```python
from build123d import *

# Parameters (mm, degrees)
SKETCH_1_W               = 26.5
SKETCH_1_H               = 26.5
SKETCH_1_R               = 9.25
EXTRUDE_1_DEPTH          = 7.5
SKETCH_3_R               = 1.75
CUT_EXTRUDE_1_DEPTH      = 14.25
CUT_EXTRUDE_1_DEPTH_BACK = 14.25


with BuildPart() as part:
    # ｽｹｯﾁ1 → ﾎﾞｽ - 押し出し1 (new body, symmetric)
    with BuildSketch(Plane.XY):
        Rectangle(SKETCH_1_W, SKETCH_1_H)
        Circle(SKETCH_1_R, mode=Mode.SUBTRACT)
    extrude(amount=EXTRUDE_1_DEPTH, both=True)

    # ｽｹｯﾁ3 → ｶｯﾄ - 押し出し1 (cut, two sides)
    with BuildSketch(Plane(origin=(0, 0, 0), x_dir=(0, 0, -1), z_dir=(1, 0, 0))) as cut_extrude_1_sk:
        Circle(SKETCH_3_R)
    extrude(amount=CUT_EXTRUDE_1_DEPTH, mode=Mode.SUBTRACT)
    extrude(cut_extrude_1_sk.sketch, amount=-CUT_EXTRUDE_1_DEPTH_BACK, mode=Mode.SUBTRACT)


solid = part.part
```
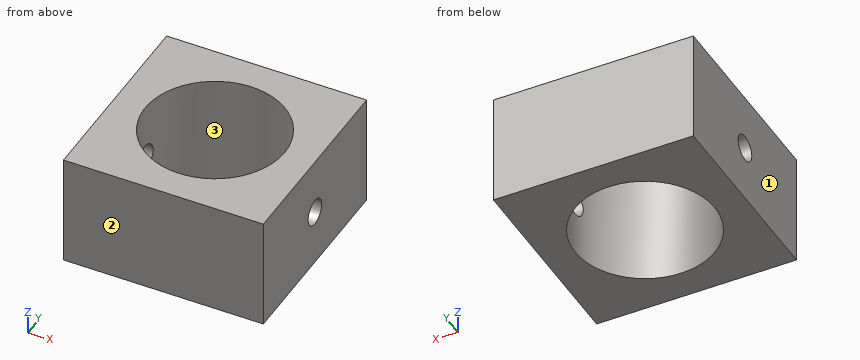
Could you check a few things on this model? Use its own coordinates, in mm. Face numbers are marked on the shaded views. Round coordinates to 2 decimals unless told otherwise and drop trailing zeros. Loops run counter-clockwise (first coordinate to the right, second up) from the corner with the lowest first, then second, coordinate; pieces in that order, holes last. Notation, with made-up numbers: (47.25, 74.5) - (56.25, 74.5) arc R14 cw to (56.25, 93.5) - close; hole circle Ø1 at (-11, 44). An arc over 180 degrees is marked (long way). Answer as CSV lines item,"result".
1. I want a section at C-C on x = 10. List the corners of the cut face in (y, z) for me, then the cut area to 3 significant figures.
Filled in:
outline,"(-13.25, -7.5) - (13.25, -7.5) - (13.25, 7.5) - (-13.25, 7.5) - close; hole circle Ø3.5 at (0, 0)"
area,"388 mm^2"
2. I want a section at B-B on y = 0. List the corners of the cut face in (x, z) for me, then the cut area to 3 significant figures.
Filled in:
outline,"(-13.25, -7.5) - (-9.25, -7.5) - (-9.25, -1.75) - (-13.25, -1.75) - close; (-13.25, 1.75) - (-9.25, 1.75) - (-9.25, 7.5) - (-13.25, 7.5) - close; (9.25, -7.5) - (13.25, -7.5) - (13.25, -1.75) - (9.25, -1.75) - close; (9.25, 1.75) - (13.25, 1.75) - (13.25, 7.5) - (9.25, 7.5) - close"
area,"92.0 mm^2"
3. Please list where these lines run through material, in increasing order: line 1 along Y through (x, z) = (0, 3.5); line 2 along Y through (x, z) = (-12.4, 0); line 3 along Z through (x, y) = (12.15, 0). Write a range as [from, to].
Filled in:
line 1,"y = [-13.25, -9.25], [9.25, 13.25]"
line 2,"y = [-13.25, -1.75], [1.75, 13.25]"
line 3,"z = [-7.5, -1.75], [1.75, 7.5]"
4. I want a section at A-A on z = 0. List the corners of the cut face in (x, y) for me, then the cut area to 3 significant figures.
Filled in:
outline,"(-13.25, -13.25) - (13.25, -13.25) - (13.25, -1.75) - (9.08, -1.75) arc R9.25 cw to (-9.08, -1.75) - (-13.25, -1.75) - close; (-13.25, 1.75) - (-9.08, 1.75) arc R9.25 cw to (9.08, 1.75) - (13.25, 1.75) - (13.25, 13.25) - (-13.25, 13.25) - close"
area,"405 mm^2"
5. For pin 1 Ø2 at (y, z) = (0, 0) entering from -X; pin 2 Ø5.5 at (y, z) = (0, 0) entering from -X, each with a flat end and sliding along its axis, tell me the tip position at first contact or that it passes through.
Filled in:
pin 1,"passes through"
pin 2,"stops at x = -13.25"
6. I want a section at D-D on y = -6. List the corners of the cut face in (x, z) for me, then the cut area to 3 significant figures.
Filled in:
outline,"(-13.25, -7.5) - (-7.04, -7.5) - (-7.04, 7.5) - (-13.25, 7.5) - close; (7.04, -7.5) - (13.25, -7.5) - (13.25, 7.5) - (7.04, 7.5) - close"
area,"186 mm^2"
7. We'd pull the mould along X, two halves only. Please class the marked faces 1, 2 and 3: +X half, -X half, draft (parallel to the pull), parting line (faces both ways), or undercut.
Filled in:
face 1,"-X half"
face 2,"draft"
face 3,"undercut"
